from build123d import *

# Parameters (mm, degrees)
F1_DEPTH = 3.175
F2_R     = 3.175


with BuildPart() as f1:
    # F0 (on Front) → F1 (new body)
    with BuildSketch(Plane.XZ):
        with BuildLine():
            Line((88.979729, -1.161793), (41.354729, -1.161793))
            Line((41.354729, -1.161793), (41.354729, -7.511793))
            ThreePointArc((41.354729, -7.511793), (43.599793, -8.441729), (44.529729, -10.686793))
            ThreePointArc((44.529729, -10.686793), (41.354729, -13.861793), (38.179729, -10.686793))
            Line((38.179729, -10.686793), (31.829729, -10.686793))
            Line((31.829729, -10.686793), (31.829729, -20.211793))
            Line((31.829729, -20.211793), (79.454729, -20.211793))
            Line((79.454729, -20.211793), (79.454729, -13.861793))
            ThreePointArc((79.454729, -13.861793), (77.209664, -8.441729), (82.629729, -10.686793))
            Line((82.629729, -10.686793), (88.979729, -10.686793))
            Line((88.979729, -10.686793), (88.979729, -1.161793))
        make_face()
        with BuildLine():
            Line((41.354729, -1.161793), (31.829729, -1.161793))
            Line((31.829729, -1.161793), (31.829729, -10.686793))
            Line((31.829729, -10.686793), (38.179729, -10.686793))
            ThreePointArc((38.179729, -10.686793), (39.109664, -8.441729), (41.354729, -7.511793))
            Line((41.354729, -7.511793), (41.354729, -1.161793))
        make_face()
        with BuildLine():
            Line((88.979729, -20.211793), (88.979729, -10.686793))
            Line((88.979729, -10.686793), (82.629729, -10.686793))
            ThreePointArc((82.629729, -10.686793), (81.699793, -12.931858), (79.454729, -13.861793))
            Line((79.454729, -13.861793), (79.454729, -20.211793))
            Line((79.454729, -20.211793), (88.979729, -20.211793))
        make_face()
    extrude(amount=F1_DEPTH)

    # F2
    f2_edges = [f1.edges().sort_by_distance(p)[0] for p in [
        (31.829729, -1.5875, -1.161793),
        (31.829729, -1.5875, -20.211793),
        (88.979729, -1.5875, -20.211793),
        (88.979729, -1.5875, -1.161793),
    ]]
    fillet(f2_edges, radius=F2_R)


solid = f1.part
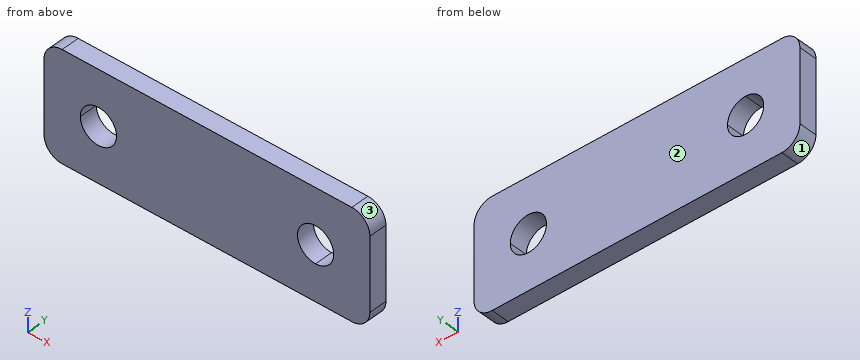
Read the model definition and answer for the solid it produces. Units are mm, in the model's axes. Face numbers are marked on the shaded views. Round coordinates to 2 decimals unless told otherwise and drop trailing zeros. Write each loop counter-clockwise with the first axis right and the second up, starting at its lowest first coordinate (ties: lowest second). Pieces come first, ordered by that corner, then holes. Notation, with made-up numbers: M 82.5,53.25 L 107.5,53.25 A37 ccw 107.5,92.25 Z; hole C -26,-24.5 d7. An arc over 180 degrees is marked long. Use a Markdown table: item, result.
1) The part is cut by section B-B (z = -12.5). Write down the section's boundary in (x, y) (3 decimals).
Answers follow:
| item | result |
|---|---|
| outline | M 31.83,-3.175 L 38.748,-3.175 L 38.748,0 L 31.83,0 Z; M 43.961,-3.175 L 76.848,-3.175 L 76.848,0 L 43.961,0 Z; M 82.061,-3.175 L 88.98,-3.175 L 88.98,0 L 82.061,0 Z |
2) For a pull along Z with two mould halves and no side action, classify the marked faces 1, 2 and 3 as pulls with the +Z half, pulls with the -Z half, needs draft (parallel to the pull), parting line crosses it, or undercut.
Answers follow:
| item | result |
|---|---|
| face 1 | pulls with the -Z half |
| face 2 | needs draft |
| face 3 | pulls with the +Z half |
3) Straight lines are drawn through the part: line 1 along X through (y, z) = (-1.5, -8.5); line 2 along X through (y, z) = (-2.45, -13.5); line 3 along X through (y, z) = (-2.1, -18.5). For each, find the intervals that lie inside material, in ascending order. Write a range as [from, to].
Answers follow:
| item | result |
|---|---|
| line 1 | x = [31.83, 39.05], [43.66, 77.15], [81.76, 88.98] |
| line 2 | x = [31.83, 39.88], [42.83, 77.98], [80.93, 88.98] |
| line 3 | x = [32.19, 88.62] |
4) The part is cut by section A-A (y = -1.35). Write down the section's boundary in (x, z) (3 decimals).
Answers follow:
| item | result |
|---|---|
| outline | M 31.83,-17.037 A3.175 ccw 35.005,-20.212 L 85.805,-20.212 A3.175 ccw 88.98,-17.037 L 88.98,-4.337 A3.175 ccw 85.805,-1.162 L 35.005,-1.162 A3.175 ccw 31.83,-4.337 Z; hole M 38.18,-10.687 A3.175 ccw long 41.355,-7.512 A3.175 ccw Z; hole M 79.455,-13.862 A3.175 ccw 82.63,-10.687 A3.175 ccw long Z |
